from build123d import *

# Parameters (mm, degrees)
BOSS_EXTRUDE1_DEPTH = 540


with BuildPart() as part:
    # Sketch1 → Boss-Extrude1 (new body)
    with BuildSketch(Plane.XY):
        Polygon((-45, -7.5), (-17.5, -7.5), (-17.5, -5), (-20, -5), (-20, 0), (-17.5, 0), (-17.5, 2.5), (-12.5, 2.5), (-12.5, 0), (-10, 0), (-10, -5), (-12.5, -5), (-12.5, -7.5), (12.5, -7.5), (12.5, -5), (10, -5), (10, 0), (12.5, 0), (12.5, 2.5), (17.5, 2.5), (17.5, 0), (20, 0), (20, -5), (17.5, -5), (17.5, -7.5), (45, -7.5), (45, -2.5), (42.5, -2.5), (42.5, -5), (37.5, -5), (37.5, 5), (42.5, 5), (42.5, 2.5), (45, 2.5), (45, 7.5), (32.5, 7.5), (32.5, 5), (35, 5), (35, 0), (32.5, 0), (32.5, -2.5), (27.5, -2.5), (27.5, 0), (25, 0), (25, 5), (27.5, 5), (27.5, 7.5), (2.5, 7.5), (2.5, 5), (5, 5), (5, 0), (2.5, 0), (2.5, -2.5), (-2.5, -2.5), (-2.5, 0), (-5, 0), (-5, 5), (-2.5, 5), (-2.5, 7.5), (-27.5, 7.5), (-27.5, 5), (-25, 5), (-25, 0), (-27.5, 0), (-27.5, -2.5), (-32.5, -2.5), (-32.5, 0), (-35, 0), (-35, 5), (-32.5, 5), (-32.5, 7.5), (-45, 7.5), (-45, 2.5), (-42.5, 2.5), (-42.5, 5), (-37.5, 5), (-37.5, -5), (-42.5, -5), (-42.5, -2.5), (-45, -2.5), align=None)
    extrude(amount=BOSS_EXTRUDE1_DEPTH)


solid = part.part
Design review of the part built by this model. Coordinates are the model's own, in mm. A direction names the side the tool comes from. Round coordinates to 2 decimals unless told otherwise and drop trailing zeros. Answer as CSV lines item,"result". Start each with the question number.
1) Tool access review of faces 4 (the face through (15, 7.5, 266)), 5 (the face through (37.5, 0, 266)): name each direction out of +Z, -Z, +X, -X, +Y, -Y from which nothing blocks a thin tool from reaching the whole face with its end or side.
2) Wall thickness on line 1 along X through (y, z) = (-2.75, 163); line 2 along X through (y, z) = (-0.25, 157.5); line 3 along X through (y, z) = (6.5, 262): over which ranges is each line inside the solid? List them lowest first. Write a range as [from, to].
3) For pin 1 Ø1.5 at (x, z) = (14, 186.5) entering from -Y; pin 2 Ø2 at (x, y) = (32.5, 2.5) entering from +Z, all flat-tipped, find the tip position at first contact; note any pin that passes through.
4) The part is to be moulded in two halves that separate along Y. For faces 1 (the face through (39, 7.5, 266)), 2 (the face through (-37.5, 0, 266)), 3 (the face through (-1, -3, 0)), say which applies: +Y half, -Y half, draft (parallel to the pull), parting line (faces both ways), or undercut.
Resolved:
1,face 4,"+Z, -Z, +X, -X, +Y"
1,face 5,"+Z, -Z"
2,line 1,"[-45, -42.5], [-37.5, -20], [-10, 10], [20, 37.5], [42.5, 45]"
2,line 2,"[-37.5, -32.5], [-27.5, -20], [-10, -2.5], [2.5, 10], [20, 27.5], [32.5, 37.5]"
2,line 3,"[-45, -32.5], [-27.5, -2.5], [2.5, 27.5], [32.5, 45]"
3,pin 1,"y = 2.5"
3,pin 2,"through"
4,face 1,"+Y half"
4,face 2,"undercut"
4,face 3,"draft"
